Autodesk Inventor part; units mm, degrees
ref_plane "YZ Plane" through (0, 0, 0) normal (1, 0, 0) x (0, 1, 0)
ref_plane "XZ Plane" through (0, 0, 0) normal (0, 1, 0) x (-1, 0, 0)
ref_plane "XY Plane" through (0, 0, 0) normal (0, 0, 1) x (1, 0, 0)
sketch "ギア線図" plane through (0, 0, 0) normal (0, 0, 1) x (1, 0, 0)
  circle A0 centre (11.2246, -29.111) radius 11.1
  circle A1 centre (54.3074, -26.8895) radius 20.05
  circle A2 centre (54.3074, -26.8895) radius 4.55
  circle A3 centre (35.8191, -9.9133) radius 11.1
  circle A4 centre (39.3074, -43.38) radius 2.05
  circle A5 centre (69.3074, -43.38) radius 2.05
  circle A6 centre (72.141, -13.5141) radius 2.05
  circle A7 centre (39.3074, -43.38) radius 15
  circle A8 centre (69.3074, -43.38) radius 15
  circle A9 centre (72.141, -13.5141) radius 15
  circle A10 centre (54.3074, -26.8895) radius 5.5 construction
  circle A11 centre (11.2246, -29.111) radius 13 construction
  circle A12 centre (54.3074, -26.8895) radius 20.5 construction
  circle A13 centre (35.8191, -9.9133) radius 20.55
  circle A14 centre (35.8191, -9.9133) radius 21.5 construction
  circle A15 centre (35.8191, -9.9133) radius 13 construction
  circle A16 centre (39.3074, -43.38) radius 2.5 construction
  circle A17 centre (69.3074, -43.38) radius 2.5 construction
  circle A18 centre (72.141, -13.5141) radius 2.5 construction
  circle A19 centre (11.2246, -29.111) radius 20.1
  circle A20 centre (11.2246, -29.111) radius 22 construction
  line L0 (39.3074, -43.38) -> (69.3074, -43.38)
  circle A21 centre (0, 0) radius 20.1
  circle A22 centre (0, 0) radius 22 construction
  circle A23 centre (39.3074, -43.38) radius 9.5 construction
  circle A24 centre (69.3074, -43.38) radius 9.5 construction
  circle A25 centre (72.141, -13.5141) radius 9.5 construction
  point P0 (58.2233, -20.0465)
  point P1 (42.0436, -35)
  point P2 (21.5995, 15.2696)
  point P3 (38.2329, 5.9161)
  point P4 (24.1755, 8.4229)
  point P5 (21.6039, 15.1272)
  point P6 (23.3458, 16.3469)
  point P7 (23.3177, 16.3886)
  dimension "d7" = 22.2
  dimension "d8" = 40.1
  dimension "d9" = 9.1
  dimension "d11" = 22.2
  dimension "d12" = 4.1
  dimension "d13" = 4.1
  dimension "d14" = 4.1
  dimension "d15" = 30
  dimension "d16" = 30
  dimension "d17" = 30
  dimension "d18" = 11
  dimension "d21" = 26
  dimension "d29" = 41
  dimension "d39" = 22.2921
  dimension "d40" = 22.2921
  dimension "d41" = 22.2921
  dimension "d43" = 41.1
  dimension "d44" = 43
  dimension "d45" = 26
  dimension "d46" = 5
  dimension "d47" = 5
  dimension "d48" = 5
  dimension "d49" = 40.2
  dimension "d50" = 44
  dimension "d53" = 40.2
  dimension "d55" = 44
  dimension "d58" = 19
  dimension "d59" = 19
  dimension "d60" = 19
sketch "スケッチ3" plane through (0, 0, 0) normal (0, 0, 1) x (1, 0, 0)
  circle A0 centre (11.2246, -29.111) radius 20.1 construction
  circle A1 centre (39.3074, -43.38) radius 15 construction
  circle A2 centre (69.3074, -43.38) radius 15 construction
  circle A3 centre (72.141, -13.5141) radius 15 construction
  circle A4 centre (11.2246, -29.111) radius 5
  circle A5 centre (59.3303, 1.1874) radius 1.5
  circle A6 centre (23.1948, 12.8161) radius 1.5
  circle A7 centre (10.6068, -54.0855) radius 1.5
  circle A8 centre (59.3303, 1.1874) radius 4.5 construction
  circle A9 centre (35.8191, -9.9133) radius 21.5 construction
  circle A10 centre (23.1948, 12.8161) radius 4.5 construction
  circle A11 centre (0, 0) radius 22 construction
  line L0 (18.6948, -58.38) -> (25.9736, -24.111)
  line L1 (25.9736, -24.111) -> (63.6708, 0)
  line L2 (63.6708, 17.3161) -> (-0.523, 17.3161)
  line L3 (-0.523, 17.3161) -> (-0.523, -58.38)
  line L4 (-0.523, -58.38) -> (18.6948, -58.38)
  line L5 (63.6708, 17.3161) -> (63.6708, 0)
  circle A12 centre (0, 0) radius 7.5
  circle A13 centre (0, 0) radius 11.5
  point P0 (-0.523, -11.4881)
  point P1 (-0.523, 11.4881)
  dimension "d69" = 9
  dimension "d61" = 10
  dimension "d63" = 3
  dimension "d64" = 3
  dimension "d67" = 3
  dimension "d70" = 9
  dimension "d71" = 15
  dimension "d72" = 4
extrude "押し出し1" add sketch "スケッチ3" along normal blind 3 contours L4 L3 A13 L2 L5 L1 L0 | A13 L3 A12 | L3 A12 A13
sketch "スケッチ4" plane through (0, 0, 3) normal (0, 0, 1) x (1, 0, 0)
  circle A0 centre (23.1948, 12.8161) radius 1.5
  circle A1 centre (59.3303, 1.1874) radius 1.5
  circle A2 centre (11.2246, -29.111) radius 5
  circle A3 centre (10.6068, -54.0855) radius 1.5
  point P0 (0, 0)
equation "\"d40\" = d39"
equation "\"d41\" = d40"
properties part number "アームフレーム" material "アルミニウム 2014-T4"
Could you check a few things on this model? Use its own coordinates, in mm. A direction names the side the tool comes from. Coordinates: 2 decimals unless noted, no trailing zeros. Loops run counter-clockwise (first coordinate to the right, second up) from the corner with the lowest first, then second, coordinate; pieces in that order, holes last. Notation, with made-up numbers: (69, -5) -> (86, -5) arc R11 cw to (86, 15) -> close; hole circle Ø5 at (48, 55.5). An arc over 180 degrees is marked (long way). Answer in a Markdown table with one row per item.
(1) Imagine slicing it at C-C (x = 15). List the corners of the cut face in (y, z) for me.
Results found:
| item | result |
|---|---|
| outline | (-58.38, 0) -> (-32.39, 0) -> (-32.39, 3) -> (-58.38, 3) -> close; (-25.83, 0) -> (17.32, 0) -> (17.32, 3) -> (-25.83, 3) -> close |
(2) For faces 4 (the face through (-0.523, -35, 1)), 5 (the face through (-0.523, 14, 1)), 6 (the face through (21.696, 12.75, 1.479)), which set-ups out of +Z, -Z, +X, -X, +Y, -Y let a thin tool reach every point of the face, with its end or its side?
Results found:
| item | result |
|---|---|
| face 4 | +Z, -Z, -X, -Y |
| face 5 | +Z, -Z, -X, +Y |
| face 6 | +Z, -Z |
(3) Will these pins go through, and if not, where does the flat tip stop? pin 1 Ø1.8 at (x, y) = (10.61, -54.09) entering from -Z; pin 2 Ø1.5 at (y, z) = (13.5, 1) entering from -X; pin 3 Ø1 at (y, z) = (-46.5, 2) entering from +X.
Results found:
| item | result |
|---|---|
| pin 1 | passes through |
| pin 2 | stops at x = -0.52 |
| pin 3 | stops at x = 21.32 |
(4) Imagine slicing it at B-B (z = 2). List the corners of the cut face in (x, y) for me, plus the area to 3 significant figures.
Results found:
| item | result |
|---|---|
| outline | (-0.52, -58.38) -> (18.69, -58.38) -> (25.97, -24.11) -> (63.67, 0) -> (63.67, 17.32) -> (-0.52, 17.32) -> (-0.52, 11.49) arc R11.5 ccw to (-0.52, -11.49) -> close; hole circle Ø15 at (0, 0); hole circle Ø10 at (11.22, -29.11); hole circle Ø3 at (10.61, -54.09); hole circle Ø3 at (23.19, 12.82); hole circle Ø3 at (59.33, 1.19) |
| area | 2,910 mm^2 |
(5) If I drill on probe 1 along Y at (x, z) = (0, 2.25); probe 2 along X at (y, z) = (-4.5, 1.35); probe 3 along Y at (x, z) = (-5, 1.05), over which ranges is the centre line in solid material (lowest first)?
Results found:
| item | result |
|---|---|
| probe 1 | y = -58.38 to -7.5, 7.5 to 17.32 |
| probe 2 | x = -10.58 to -6, 6 to 56.64 |
| probe 3 | y = -10.36 to -5.59, 5.59 to 10.36 |
(6) Imagine slicing it at A-A (y = -32.5). List the corners of the cut face in (x, z) for me.
Results found:
| item | result |
|---|---|
| outline | (-0.52, 0) -> (7.55, 0) -> (7.55, 3) -> (-0.52, 3) -> close; (14.9, 0) -> (24.19, 0) -> (24.19, 3) -> (14.9, 3) -> close |
(7) Thinking about a two-plate mould opening in Y: for faces 1 (the face through (32, 17.316, 1)), 2 (the face through (13.91, -33.33, 1.48)), 3 (the face through (9, -58.38, 1)), which applies, released by +Y, released by -Y, zero draft, split by the parting line, or undercut?
Results found:
| item | result |
|---|---|
| face 1 | released by +Y |
| face 2 | undercut |
| face 3 | released by -Y |
(8) Imagine slicing it at D-D (x = 30.5). List the corners of the cut face in (y, z) for me.
Results found:
| item | result |
|---|---|
| outline | (-21.22, 0) -> (17.32, 0) -> (17.32, 3) -> (-21.22, 3) -> close |
